Build history of the part. All positions in model axes, mm. Face numbers are marked on the shaded views. Coordinates: 2 decimals unless noted, no trailing zeros. Loops run counter-clockwise (first coordinate to the right, second up) from the corner with the lowest first, then second, coordinate; pieces in that order, holes last.
Item 1: Mould opens along Z. For the marked faces 1, 2 and 3 say: released by +Z, released by -Z, zero draft, split by the parting line, or undercut.
Item 2: Drill centre lines: line 1 along Z through (x, y) = (16.25, 0); line 2 along Z through (x, y) = (4.75, 1.5). Where is each one in solid material? Low to high.
Item 3: Flat gauge pins, fed straight in: pin 1 (1.5 mm diameter, centred on x = 5.5, z = 5.5, fed in from -Y); pin 2 (1.5 mm diameter, centred on x = 2.5, y = 1, fed in from +Z); pin 3 (1.5 mm diameter, centred on x = 11, z = -6.5, fed in from +Y). Where does each tip first touch, or does it go through?
Item 4: Cut at C-C (x = 4). List the corners of the cut face in (y, z), and give its area (3 significant figures).
from build123d import *

# Parameters (mm, degrees)
F0_W = 20
F0_H = 4
F4_R = 1.99999


# Not quite as in the source:
# - a fillet or chamfer is up to 0.001 mm smaller than in the source, because OpenCascade refuses the exact size


with BuildPart() as f1:
    # F0 (on Front) → F1 (revolve)
    with BuildSketch(Plane.XZ):
        with Locations((10, 9)):
            Rectangle(F0_W, F0_H)
    revolve(axis=Axis((12.6487514935, 0, 0), (1, 0, 0)))

    # F2 (on Front) → F3 (revolve, cut)
    with BuildSketch(Plane.XZ):
        Polygon((24, 11.9697983939), (13, 11.9697983939), (24, 10.0302016061), align=None)
    revolve(axis=Axis((11.270377785, 0, 0), (1, 0, 0)), mode=Mode.SUBTRACT)

    # F4 (radius 2 in the source; OpenCascade refuses exactly that, so slightly less here)
    f4_edges = [f1.edges().sort_by_distance(p)[0] for p in [
        (0, 0, -11),
        (0, 0, -7),
    ]]
    fillet(f4_edges, radius=F4_R)


solid = f1.part
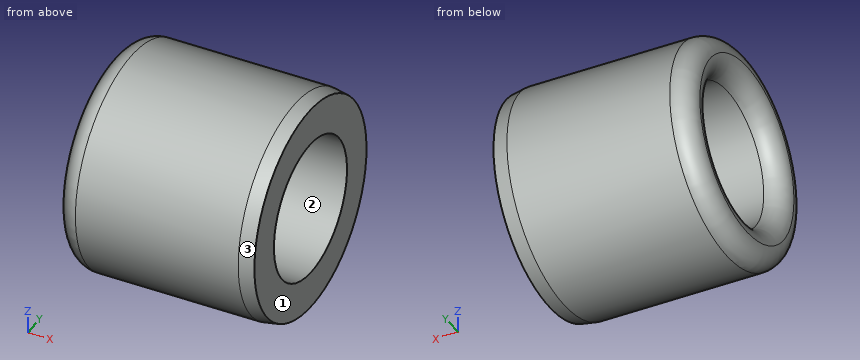
Filled sheet:
1. face 1: zero draft
1. face 2: undercut
1. face 3: split by the parting line
2. line 1: z = -11 to -7, 7 to 11
2. line 2: z = -10.9 to -6.84, 6.84 to 10.9
3. pin 1: stops at y = -9.92
3. pin 2: stops at z = 11
3. pin 3: stops at y = 9.38
4. outline: circle Ø22 at (0, 0); hole circle Ø14 at (0, 0)
4. area: 226 mm2
